```python
from build123d import *

# Parameters (mm, degrees)
SKETCH1_W           = 4.09
SKETCH1_H           = 3.02
BOSS_EXTRUDE1_DEPTH = 3.02
SKETCH2_R           = 0.1075
BOSS_EXTRUDE2_DEPTH = 15.25


with BuildPart() as part:
    # Sketch1 → Boss-Extrude1 (new body)
    with BuildSketch(Plane.XY):
        with Locations((2.045, 1.51)):
            Rectangle(SKETCH1_W, SKETCH1_H)
    extrude(amount=BOSS_EXTRUDE1_DEPTH)

    # Sketch2 → Boss-Extrude2 (add)
    with BuildSketch(Plane(origin=(0, 3.02, 0), x_dir=(1, 0, 0), z_dir=(0, 1, 0))):
        with Locations(Location((0.775, -1, 0), (0, 0, 270))):
            Circle(SKETCH2_R)
        with Locations(Location((2.045, -1, 0), (0, 0, 270))):
            Circle(SKETCH2_R)
        with Locations(Location((3.315, -1, 0), (0, 0, 270))):
            Circle(SKETCH2_R)
    extrude(amount=BOSS_EXTRUDE2_DEPTH)


solid = part.part
```
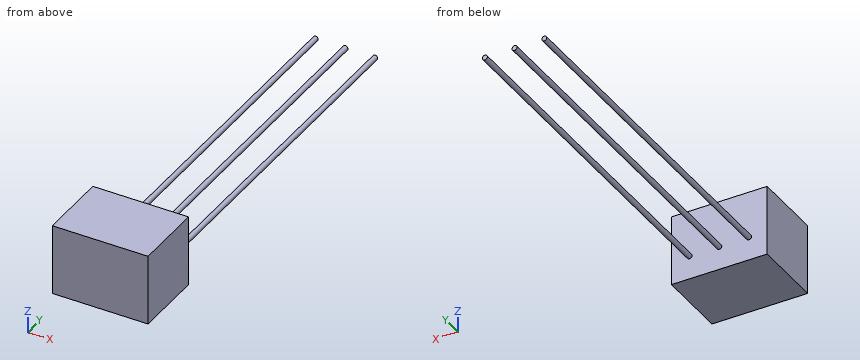
Check sheet for the modelled part. Datum: model origin and axes. Units: mm. Coordinates: 2 decimals unless noted, no trailing zeros. Write each loop counter-clockwise with the first axis right and the second up, starting at its lowest first coordinate (ties: lowest second). Pieces come first, ordered by that corner, then holes. Notation, with made-up numbers: (72.25, 33.5) -> (109.25, 33.5) arc R24 cw to (109.25, 68.5) -> close; hole circle Ø8 at (80, 32). An arc over 180 degrees is marked (long way). Use a Markdown table: item, result.
1. Sectioned sample at A-A (x = 1.6). Enter the section's corners in (y, z).
Reported:
| item | result |
|---|---|
| outline | (0, 0) -> (3.02, 0) -> (3.02, 3.02) -> (0, 3.02) -> close |
2. Sectioned sample at B-B (z = 1.9). Enter the section's corners in (x, y).
Reported:
| item | result |
|---|---|
| outline | (0, 0) -> (4.09, 0) -> (4.09, 3.02) -> (0, 3.02) -> close |
3. Sectioned sample at C-C (y = 5). Enter the section's corners in (x, z) (1 decimal), plus the area to 3 significant figures.
Reported:
| item | result |
|---|---|
| outline | circle Ø0.2 at (0.8, 1); circle Ø0.2 at (2, 1); circle Ø0.2 at (3.3, 1) |
| area | 0.109 mm2 |
4. Go/stop test with a flat-tipped pin: pin 1 Ø0.9 at (x, z) = (2.5, 2) entering from +Y. Record where the tip stops, or that it passes through.
Reported:
| item | result |
|---|---|
| pin 1 | stops at y = 3.02 |
5. Scan lines: line 1 along X through (y, z) = (12.75, 1); line 2 along Y through (x, z) = (1.85, 1.05); line 3 along Z through (x, y) = (3.3, 13.75). Record each from-to range of solid material in increasing order.
Reported:
| item | result |
|---|---|
| line 1 | x = 0.67 to 0.88, 1.94 to 2.15, 3.21 to 3.42 |
| line 2 | y = 0 to 3.02 |
| line 3 | z = 0.89 to 1.11 |
